Source: CAD feature listing. Evaluate the final solid. Frame: model axes, mm. A direction names the side the tool comes from. Round coordinates to 2 decimals unless told otherwise and drop trailing zeros. Order: outer loops, then holes, each group sorted by start corner. A loop starts at its lowest first (then second) coordinate and runs counter-clockwise, first axis right, second up. Notation, with made-up numbers: (71.5, -8.5) - (103.5, -8.5) arc R17 ccw to (103.5, 18.5) - close; hole circle Ø1 at (31.25, 58.5). An arc over 180 degrees is marked (long way). Use one line per item in the form item = value. Start each with the question number.
Q1. Cut plane C-C, the plane z = -9.5. Return the cut outline in (x, y).
Q2. Pin query (flat end, axial travel): pin 1 Ø2 at (y, z) = (11, -40) entering from -X; pin 2 Ø1.2 at (x, z) = (75, -25) entering from -Y; pin 3 Ø20 at (x, z) = (-101, 10) entering from +Y. Return the tip coordinate at first contact, or that it passes through.
Q3. Cut plane A-A, the plane y = 31. Return the cut outline in (x, z).
Q4. Draft query along Y for faces 6 (the flat face through (75, 5, -25)), 7 (the cylindrical face through (-73, 2, 25)), 8 (the flat face through (20, 11, 55)). Return one class per face: released by +Y, released by -Y, zero draft, split by the parting line, or undercut.
Q5. Set-up query: faces 1 (the flat face through (20, 19, 55)), 2 (the flat face through (-75, 5, 25)), 3 (the flat face through (-2, 25, 57.5)), 4 (the flat face through (-89.5, 30, 1)), 5 (the flat face through (107.5, 25, 1)). Return all of +Z, -Z, +X, -X, +Y, -Y with unobstructed straight access to the full face (end or side cutting, diameter ignored); none if empty.
Q6. Cut plane B-B, the plane z = 25. Return the cut outline in (x, y).
Q7. Ray query, line 1 (X direction, y = 1.95, z = -25); line 2 (Z direction, x = -97.5, y = 34.5); line 3 (X direction, y = 21.5, z = -4). Return the intervals inside material, ascending. Write a range as [from, to].
from build123d import *

# Parameters (mm, degrees)
SKETCH1_W           = 215
SKETCH1_H           = 115
BOSS_EXTRUDE1_DEPTH = 50
SKETCH2_W           = 18
SKETCH2_H           = 111.5
CUT_EXTRUDE1_DEPTH  = 41.25
SKETCH3_R           = 2
CUT_EXTRUDE2_DEPTH  = 5
SKETCH4_W           = 15
SKETCH4_H           = 8
CUT_EXTRUDE3_DEPTH  = 5


with BuildPart() as part:
    # Sketch1 → Boss-Extrude1 (new body)
    with BuildSketch(Plane(origin=(0, 0, 0), x_dir=(1, 0, 0), z_dir=(0, 1, 0))):
        Rectangle(SKETCH1_W, SKETCH1_H)
    extrude(amount=BOSS_EXTRUDE1_DEPTH)

    # Sketch2 → Cut-Extrude1 (cut)
    with BuildSketch(Plane(origin=(0, 50, 0), x_dir=(1, 0, 0), z_dir=(0, 1, 0))):
        with Locations((-98.5, 0)):
            Rectangle(SKETCH2_W, SKETCH2_H)
    extrude(amount=-CUT_EXTRUDE1_DEPTH, mode=Mode.SUBTRACT)

    # Sketch3 → Cut-Extrude2 (cut)
    with BuildSketch(Plane.XZ):
        with Locations(Location((-75, -25, 0), (0, 0, 270))):  # turned: the seam where the file's is
            Circle(SKETCH3_R)
        with Locations(Location((-75, 25, 0), (0, 0, 270))):  # turned: the seam where the file's is
            Circle(SKETCH3_R)
        with Locations(Location((75, -25, 0), (0, 0, 270))):  # turned: the seam where the file's is
            Circle(SKETCH3_R)
        with Locations(Location((75, 25, 0), (0, 0, 270))):  # turned: the seam where the file's is
            Circle(SKETCH3_R)
    extrude(amount=-CUT_EXTRUDE2_DEPTH, mode=Mode.SUBTRACT)

    # Sketch4 → Cut-Extrude3 (cut)
    with BuildSketch(Plane.XY.offset(57.5)):
        with Locations((20.5, 15)):
            Rectangle(SKETCH4_W, SKETCH4_H)
    extrude(amount=-CUT_EXTRUDE3_DEPTH, mode=Mode.SUBTRACT)


solid = part.part
Completed:
q1.outline = (-107.5, 0) - (107.5, 0) - (107.5, 50) - (-89.5, 50) - (-89.5, 8.75) - (-107.5, 8.75) - close
q2.pin_1 = -89.5
q2.pin_2 = 5
q2.pin_3 = 8.75
q3.outline = (-107.5, -57.5) - (107.5, -57.5) - (107.5, 57.5) - (-107.5, 57.5) - (-107.5, 55.75) - (-89.5, 55.75) - (-89.5, -55.75) - (-107.5, -55.75) - close
q4.face_6 = released by -Y
q4.face_7 = zero draft
q4.face_8 = undercut
q5.face_1 = +Z
q5.face_2 = -Y
q5.face_3 = +Z, +X, -X, +Y, -Y
q5.face_4 = -X, +Y
q5.face_5 = +Z, -Z, +X, +Y, -Y
q6.outline = (-107.5, 0) - (-77, 0) - (-77, 5) - (-73, 5) - (-73, 0) - (73, 0) - (73, 5) - (77, 5) - (77, 0) - (107.5, 0) - (107.5, 50) - (-89.5, 50) - (-89.5, 8.75) - (-107.5, 8.75) - close
q7.line_1 = [-107.5, -77], [-73, 73], [77, 107.5]
q7.line_2 = [-57.5, -55.75], [55.75, 57.5]
q7.line_3 = [-89.5, 107.5]
